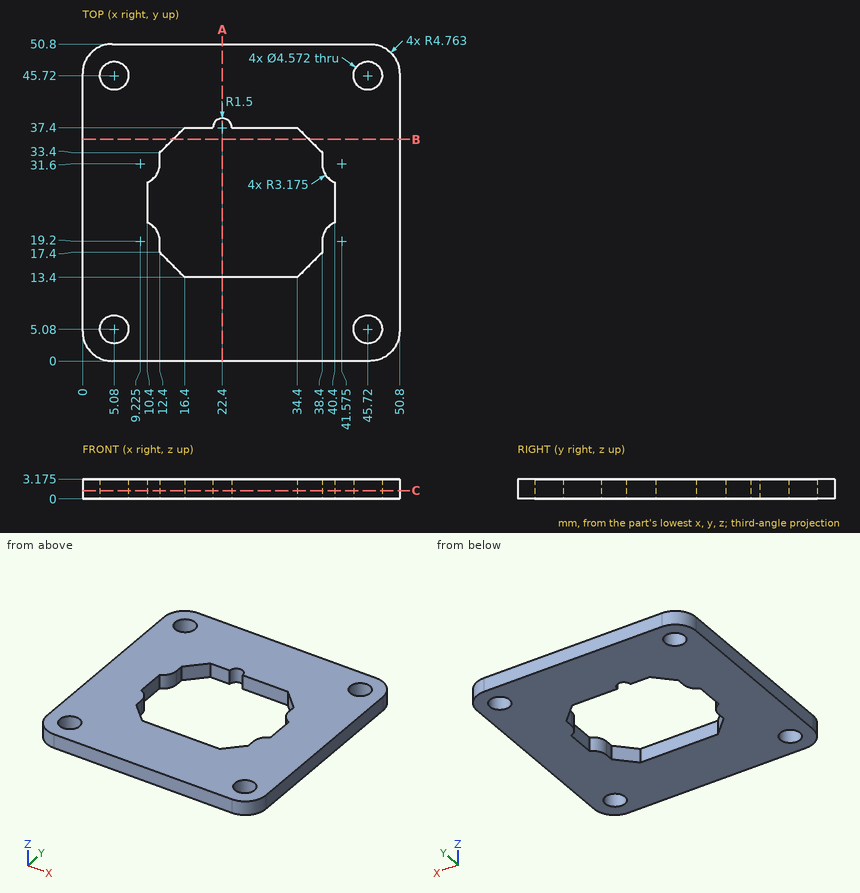
Study the drawing (mm; zero at the part's minimum x, y, z) and answer. Give positions to 0.01 mm unless a question says otherwise; leave off trailing zeros. Write each loop counter-clockwise with the first axis right and the second up, starting at its lowest first coordinate (ties: lowest second). Pieces come first, ordered by that corner, then holes.
(1) A flat-ended cylindrical pin translates along its axis: pin 1 Ø2.5 at (x, y) = (5.08, 5.08) entering from +Z. Find the tip coordinate at first contact, or state that the pin passes through.
Final values:
pin 1: passes through
(2) The part is cut by section B-B on y = 35.5. Write down the section's boundary in (x, z) (1 decimal).
Final values:
outline: (0, 0) - (14.5, 0) - (14.5, 3.2) - (0, 3.2) - close; (36.3, 0) - (50.8, 0) - (50.8, 3.2) - (36.3, 3.2) - close
(3) Straight lines are drawn through the part: line 1 (Y direction, x = 5.08, z = 1.15) (1 decimal); line 2 (Y direction, x = 30.5, z = 0.6). For each, find the intervals that lie inside material, in ascending order.
Final values:
line 1: y = 0 to 2.8, 7.4 to 43.4, 48 to 50.8
line 2: y = 0 to 13.4, 37.4 to 50.8
(4) The part is cut by section A-A on x = 22.4. Write down the section's boundary in (y, z) (1 decimal).
Final values:
outline: (0, 0) - (13.4, 0) - (13.4, 3.2) - (0, 3.2) - close; (38.9, 0) - (50.8, 0) - (50.8, 3.2) - (38.9, 3.2) - close
(5) The part is cut by section C-C on z = 1.3. Count the separate pieces of the cut face and the enclosed holes in it, plus the area to 3 significant figures.
Final values:
separate pieces: 1
enclosed holes: 5
area: 1,870 mm2
